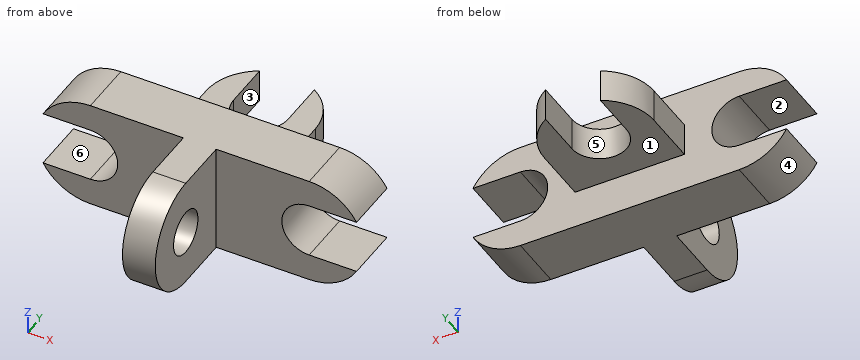
```python
from build123d import *

# Parameters (mm, degrees)
BOSS_EXTRUDE1_DEPTH = 25
SKETCH2_W           = 100
SKETCH2_H           = 30
BOSS_EXTRUDE3_DEPTH = 150
CUT_EXTRUDE1_DEPTH  = 150
BOSS_EXTRUDE4_DEPTH = 15
SKETCH7_R           = 20
CUT_EXTRUDE2_DEPTH  = 30


with BuildPart() as part:
    # Sketch1 → Boss-Extrude1 (new body, symmetric)
    with BuildSketch(Plane(origin=(0, 0, 0), x_dir=(1, 0, 0), z_dir=(0, 1, 0))):
        with BuildLine():
            Line((100, 50), (-100, 50))
            ThreePointArc((-100, 50), (-125, 43.301270189), (-143.301270189, 25))
            Line((-143.301270189, 25), (-100, 25))
            ThreePointArc((-100, 25), (-75, 0), (-100, -25))
            Line((-100, -25), (-143.301270189, -25))
            ThreePointArc((-143.301270189, -25), (-125, -43.301270189), (-100, -50))
            Line((-100, -50), (100, -50))
            ThreePointArc((100, -50), (125, -43.301270189), (143.301270189, -25))
            Line((143.301270189, -25), (100, -25))
            ThreePointArc((100, -25), (75, 0), (100, 25))
            Line((100, 25), (143.301270189, 25))
            ThreePointArc((143.301270189, 25), (125, 43.301270189), (100, 50))
        make_face()
    extrude(amount=BOSS_EXTRUDE1_DEPTH, both=True)

    # Sketch2 → Boss-Extrude3 (add)
    with BuildSketch(Plane(origin=(0, 25, 0), x_dir=(1, 0, 0), z_dir=(0, 1, 0))):
        Rectangle(SKETCH2_W, SKETCH2_H)
    extrude(amount=BOSS_EXTRUDE3_DEPTH)

    # Sketch4 → Cut-Extrude1 (cut)
    with BuildSketch(Plane.XY.offset(15)):
        with BuildLine():
            Line((-25, 75), (-25, 118.301270189))
            ThreePointArc((-25, 118.301270189), (-43.301270189, 100), (-50, 75))
            Line((-50, 75), (-50, 175))
            Line((-50, 175), (50, 175))
            Line((50, 175), (50, 75))
            ThreePointArc((50, 75), (43.301270189, 100), (25, 118.301270189))
            Line((25, 118.301270189), (25, 75))
            ThreePointArc((25, 75), (0, 50), (-25, 75))
        make_face()
    extrude(amount=-CUT_EXTRUDE1_DEPTH, mode=Mode.SUBTRACT)

    # Sketch6 → Boss-Extrude4 (add, symmetric)
    with BuildSketch(Plane(origin=(0, 0, 0), x_dir=(0, 0, -1), z_dir=(1, 0, 0))):
        with BuildLine():
            Line((-50, -74.998729811), (-50, -25))
            Line((-50, -25), (-25, -25))
            Line((-25, -25), (25, -25))
            Line((25, -25), (50, -25))
            Line((50, -25), (50, -74.998729811))
            ThreePointArc((50, -74.998729811), (0, -124.998729811), (-50, -74.998729811))
        make_face()
    extrude(amount=BOSS_EXTRUDE4_DEPTH, both=True)

    # Sketch7 → Cut-Extrude2 (cut)
    with BuildSketch(Plane(origin=(15, 0, 0), x_dir=(0, 0, -1), z_dir=(1, 0, 0))):
        with Locations((0, -74.998729811)):
            Circle(SKETCH7_R)
    extrude(amount=-CUT_EXTRUDE2_DEPTH, mode=Mode.SUBTRACT)


solid = part.part
```
Input: part model. Units: mm. Frame: model coordinates. Face numbers are marked on the shaded views. A direction names the side the tool comes from. Give positions to 0.01 mm unless a question says otherwise; leave off trailing zeros. Order: outer loops, then holes, each group sorted by start corner. A loop starts at its lowest first (then second) coordinate and runs counter-clockwise, first axis right, second up. Notation, with made-up numbers: M 55,-31 L 112,-31 A25 ccw 112,-19 Z; hole C 5.5,37.5 d10. An arc over 180 degrees is marked long. One line per question, with ' | ' between items.
1) Section D-D on x = 0. Output: boundary loops of the cut face in (y, z), and give its area (3 significant figures).
Filled in:
outline: M -75,-50 L 25,-50 L 25,-15 L 50,-15 L 50,15 L 25,15 L 25,50 L -75,50 A50 ccw Z; hole C -75,0 d40 | area: 13,400 mm2
2) Access query for the marked faces 1, 2 and 3. Directions: +Z, -Z, +X, -X, +Y, -Y. A direction counts if a zero-diameter tool reaches every point of the face in a straight line with its end or side. Return the directions, or none.
Filled in:
face 1: -Z, +X, -X, +Y | face 2: -X, +Y, -Y | face 3: +Z, -Z, +Y
3) Ray query, L1, parallel to Y at x = -0.75, z = 0; L2, parallel to X at y = 76.5, z = 5.5; L3, parallel to Y at x = -41, z = 18. Return the intervals inside material, ascending.
Filled in:
L1: y = -125 to -95, -55 to 50.01 | L2: x = -49.98 to -25, 25 to 49.98 | L3: y = -25 to 25
4) Contact query for flat-ended pins moving along their axis: P1, Ø5, axis at x = -6, z = 33.5, coming from the -Y side; P2, Ø1, axis at x = 106, y = -4, coming from the -Z side; P3, Ø1.5, axis at y = 36.5, z = -12.5, coming from the -X side; P4, Ø5, axis at y = -26, z = 25.5, coming from the -X side. Output: stop coordinate, or through.
Filled in:
P1: stops at y = -114.23 | P2: stops at z = -49.7 | P3: stops at x = -50 | P4: stops at x = -143.3
5) Draft query along Z for the marked faces 4, 5 and 6. Return one class per face: pulls with the +Z half, pulls with the -Z half, needs draft (parallel to the pull), parting line crosses it, or undercut.
Filled in:
face 4: pulls with the -Z half | face 5: needs draft | face 6: undercut
6) Section B-B on x = 107. Output: boundary loops of the cut face in (y, z), and give its area (3 significant figures).
Filled in:
outline: M -25,-49.51 L 25,-49.51 L 25,-25 L -25,-25 Z; M -25,25 L 25,25 L 25,49.51 L -25,49.51 Z | area: 2,450 mm2
7) Section A-A on z = 0. Output: boundary loops of the cut face in (x, y), and give its area (3 significant figures).
Filled in:
outline: M -75,-25 L -15,-25 L -15,-55 L 15,-55 L 15,-25 L 75,-25 L 75,25 L 50,25 L 50,75 A50 ccw 25,118.3 L 25,75 A25 cw -25,75 L -25,118.3 A50 ccw -50,75 L -50,25 L -75,25 Z; M -15,-125 L 15,-125 L 15,-95 L -15,-95 Z | area: 14,900 mm2
8) Section C-C on y = 58. Output: boundary loops of the cut face in (x, z), and give its area (3 significant figures).
Filled in:
outline: M -50,-15 L -18.33,-15 L -18.33,15 L -50,15 Z; M 18.33,-15 L 50,-15 L 50,15 L 18.33,15 Z | area: 1,900 mm2
